Read the model definition and answer for the solid it produces. Units are mm, in the model's axes. Coordinates: 2 decimals unless noted, no trailing zeros. Answer in a Markdown table with one row per item.
Autodesk Inventor part; units mm, degrees
ref_plane "Work Plane1" through (0, -20, 0) normal (0, 1, 0) x (-1, 0, 0)
ref_plane "YZ Plane" through (0, 0, 0) normal (1, 0, 0) x (0, 1, 0)
ref_plane "XY Plane" through (0, 0, 0) normal (0, 0, 1) x (1, 0, 0)
sketch "Sketch1" plane through (0, 0, 0) normal (0, 1, 0) x (-1, 0, 0)
  line L0 (552.5, 227.5) -> (-552.5, 227.5)
  line L1 (-552.5, 227.5) -> (-552.5, -227.5)
  line L2 (-552.5, -227.5) -> (552.5, -227.5)
  line L3 (552.5, -227.5) -> (552.5, 227.5)
  line L4 (552.5, 227.5) -> (-552.5, -227.5) construction
  line L5 (-552.5, 227.5) -> (552.5, -227.5) construction
  point P0 (0, 0)
  dimension "d0" = 1105
  dimension "d1" = 455
ref_plane "Work Plane1" through (0, -20, 0) normal (0, 1, 0) x (-1, 0, 0)
sketch "Sketch2" plane through (0, -20, 0) normal (0, 1, 0) x (-1, 0, 0)
  line L0 (-537.5, 212.5) -> (537.5, 212.5)
  line L1 (537.5, 212.5) -> (537.5, -212.5)
  line L2 (537.5, -212.5) -> (-537.5, -212.5)
  line L3 (-537.5, -212.5) -> (-537.5, 212.5)
  line L4 (-537.5, 212.5) -> (537.5, -212.5) construction
  line L5 (537.5, 212.5) -> (-537.5, -212.5) construction
  point P0 (0, 0)
  dimension "d3" = 1075
  dimension "d4" = 425
loft "Loft1" add profiles "Sketch1", "Sketch2"
shell "Shell1" thickness 3 removed faces 1 at (184.1667, 0, 75.8333)
properties part number "ChipTray"
Q1. For a pull along Z with two mould halves and no side action, classify faces 1 (the face through (-10, -17, -2)), 2 (the face through (-10, -20, -2)) as pulls with the +Z half, pulls with the -Z half, needs draft (parallel to the pull), parting line crosses it, or undercut.
Outcome:
| item | result |
|---|---|
| face 1 | undercut |
| face 2 | needs draft |
Q2. Consider line 1 (Y direction, x = -404, z = -141.5); line 2 (X direction, y = -4.25, z = 186.5); line 3 (Z direction, x = -94.5, y = -3). Determine where each line is inside the solid, lowest interval first.
Outcome:
| item | result |
|---|---|
| line 1 | -20 to -17 |
| line 2 | -549.31 to -545.56, 545.56 to 549.31 |
| line 3 | -225.25 to -221.5, 221.5 to 225.25 |
Q3. Given pin 1 (3 mm diameter, centred on y = -11.5, z = 47, fed in from +X); pin 2 (4 mm diameter, centred on y = -12.5, z = 138.5, fed in from +X) (3 decimals); pin 3 (5 mm diameter, centred on x = 304.5, y = -9.5, fed in from +Z), each flat-ended and moving along its own axis, determine where each tip first touches the part or whether it passes through.
Outcome:
| item | result |
|---|---|
| pin 1 | x = 545 |
| pin 2 | x = 544.625 |
| pin 3 | z = 222.25 |
